Source: CAD feature listing. Evaluate the final solid. Frame: model axes, mm. A direction names the side the tool comes from. Round coordinates to 2 decimals unless told otherwise and drop trailing zeros. Write each loop counter-clockwise with the first axis right and the second up, starting at its lowest first coordinate (ties: lowest second). Pieces come first, ordered by that corner, then holes.
```python
from build123d import *

# Parameters (mm, degrees)
F1_DEPTH = 36
F3_DEPTH = 12


with BuildPart() as f1:
    # F0 (on Front) → F1 (new body)
    with BuildSketch(Plane.XZ):
        Polygon((-30, 22.5), (-30, -22.5), (-10, -22.5), (-10, 2.5), (10, 2.5), (10, -22.5), (30, -22.5), (30, 22.5), (10, 22.5), (-10, 22.5), align=None)
    extrude(amount=F1_DEPTH)

    # F2 (on face) → F3 (join)
    with BuildSketch(Plane.XY.offset(22.5)):
        Polygon((-30, -18), (-12, 0), (-30, 0), align=None)
        Polygon((30, 0), (12, 0), (30, -18), align=None)
    extrude(amount=F3_DEPTH)


solid = f1.part
```
Q1. Mould query, pull axis X, two halves, no side actions, for faces 4 (the face through (-30, -18, 6)), 5 (the face through (0, -18, 2.5)), 6 (the face through (0, 0, 6)). Classes: pulls with the +X half, pulls with the -X half, needs draft (parallel to the pull), parting line crosses it, or undercut.
Q2. Line query: line 1 (X direction, y = -8, z = -2.5); line 2 (Z direction, x = -22, y = -16); line 3 (Z direction, x = 0, y = -17). Output: solid intervals per line, ascending.
Q3. Section query C-C, the plane x = -25. Output: boundary loops of the cut face in (y, z), and give its area (3 significant figures).
Q4. Set-up query: faces 1 (the face through (0, -22, 22.5)), 2 (the face through (-10, -18, -10)), 3 (the face through (0, -36, 5)). Return all of +Z, -Z, +X, -X, +Y, -Y with unobstructed straight access to the full face (end or side cutting, diameter ignored); none if empty.
Q5. Section query D-D, the plane y = -22.5. Output: boundary loops of the cut face in (x, z), and give its area (3 significant figures).
Q6. Section query B-B, the plane y = -3.5. Output: boundary loops of the cut face in (x, z), and give its area (3 significant figures).
Q7. Pin query (flat end, axial travel): P1, Ø4, axis at x = 1.5, y = -22, coming from the -Z side; P2, Ø10, axis at x = 22.5, y = -20.5, coming from the +Z side. Return the tip coordinate at first contact, or that it passes through.
Q8. Section query A-A, the plane z = -12.5. Output: boundary loops of the cut face in (x, y), and give its area (3 significant figures).
Filled in:
1. face 4: pulls with the -X half
1. face 5: undercut
1. face 6: needs draft
2. line 1: x = -30 to -10, 10 to 30
2. line 2: z = -22.5 to 22.5
2. line 3: z = 2.5 to 22.5
3. outline: (-36, -22.5) - (0, -22.5) - (0, 34.5) - (-13, 34.5) - (-13, 22.5) - (-36, 22.5) - close
3. area: 1,780 mm2
4. face 1: +Z, -Y
4. face 2: -Z, +Y, -Y
4. face 3: +Z, -Z, +X, -X, -Y
5. outline: (-30, -22.5) - (-10, -22.5) - (-10, 2.5) - (10, 2.5) - (10, -22.5) - (30, -22.5) - (30, 22.5) - (-30, 22.5) - close
5. area: 2,200 mm2
6. outline: (-30, -22.5) - (-10, -22.5) - (-10, 2.5) - (10, 2.5) - (10, -22.5) - (30, -22.5) - (30, 34.5) - (15.5, 34.5) - (15.5, 22.5) - (-15.5, 22.5) - (-15.5, 34.5) - (-30, 34.5) - close
6. area: 2,550 mm2
7. P1: stops at z = 2.5
7. P2: stops at z = 22.5
8. outline: (-30, -36) - (-10, -36) - (-10, 0) - (-30, 0) - close; (10, -36) - (30, -36) - (30, 0) - (10, 0) - close
8. area: 1,440 mm2
